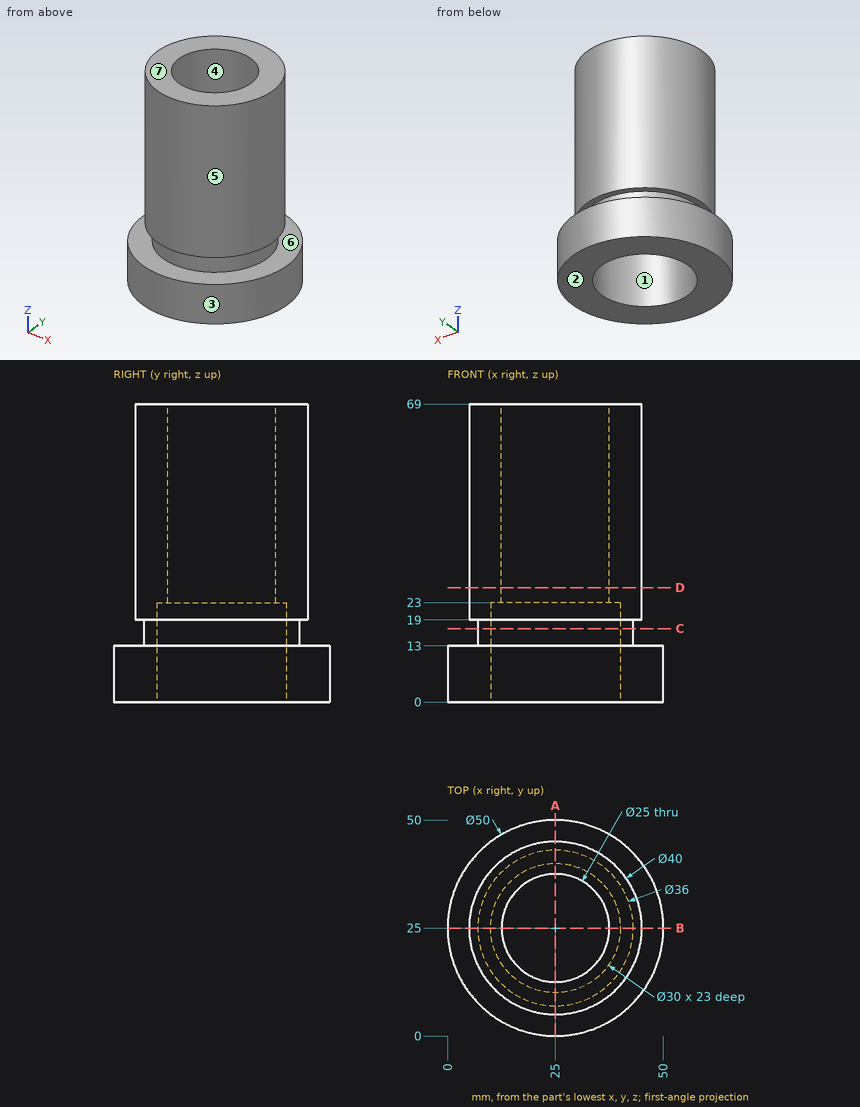
Input: dimensioned drawing with shaded views. Units: mm. Origin: part minimum x, y, z. A direction names the side the tool comes from. Coordinates: 2 decimals unless noted, no trailing zeros. Loops run counter-clockwise (first coordinate to the right, second up) from the corner with the lowest first, then second, coordinate; pieces in that order, holes last. Notation, with made-up numbers: M 46.25,64.5 L 103.25,64.5 A17 cw 103.25,75.5 Z; hole C 48,81 d4. An arc over 180 degrees is marked long. Use a Markdown table: item, result. Add a question column.
1) Section A-A, the plane x = 25. Return the cut outline in (y, z).
2) Line query: L1, parallel to Y at x = 25, z = 7; L2, parallel to Z at x = 39.5, y = 13; L3, parallel to Y at x = 25, z = 54.5. Output: solid intervals per line, ascending. Write a range as from..to.
3) Pin query (flat end, axial travel): P1, Ø3, axis at x = 15, z = 54.5, coming from the -Y side; P2, Ø5, axis at x = 18, z = 18, coming from the -Y side; P3, Ø2, axis at y = 5.5, z = 47, coming from the +X side. Return the tip coordinate at first contact, or that it passes through.
4) Section C-C, the plane z = 17. Return the cut outline in (x, y).
5) Set-up query: the marked faces 5, 6 and 7. Return all of +Z, -Z, +X, -X, +Y, -Y with unobstructed straight access to the full face (end or side cutting, diameter ignored); none if empty.
6) Section D-D, the plane z = 26.5. Return the cut outline in (x, y).
7) Draft query along X for the marked faces 1, 2, 3 and 4. Return one class per face: +X half, -X half, draft (parallel to the pull), parting line (faces both ways), or undercut.
Answer below:
| question | item | result |
|---|---|---|
| 1 | outline | M 0,0 L 10,0 L 10,23 L 12.5,23 L 12.5,69 L 5,69 L 5,19 L 7,19 L 7,13 L 0,13 Z; M 37.5,23 L 40,23 L 40,0 L 50,0 L 50,13 L 43,13 L 43,19 L 45,19 L 45,69 L 37.5,69 Z |
| 2 | L1 | 0..10, 40..50 |
| 2 | L2 | 0..13, 19..69 |
| 2 | L3 | 5..12.5, 37.5..45 |
| 3 | P1 | y = 6.9 |
| 3 | P2 | y = 5.56 |
| 3 | P3 | x = 32.6 |
| 4 | outline | C 25,25 d36; hole C 25,25 d30 |
| 5 | face 5 | +Z |
| 5 | face 6 | none |
| 5 | face 7 | +Z, +X, -X, +Y, -Y |
| 6 | outline | C 25,25 d40; hole C 25,25 d25 |
| 7 | face 1 | undercut |
| 7 | face 2 | draft |
| 7 | face 3 | parting line |
| 7 | face 4 | undercut |
